Build history of the part. All positions in model axes, mm. A direction names the side the tool comes from. Round coordinates to 2 decimals unless told otherwise and drop trailing zeros. Order: outer loops, then holes, each group sorted by start corner. A loop starts at its lowest first (then second) coordinate and runs counter-clockwise, first axis right, second up. Notation, with made-up numbers: (46, 27.25) -> (80, 27.25) arc R28 ccw to (80, 66.25) -> close; hole circle Ø1 at (49.25, 70). An arc over 180 degrees is marked (long way). Use a Markdown table: item, result. Add a question column.
Item 1: Slice it at A-A, the plane z = -3.25. Give the cut face in (x, y) (3 decimals).
Item 2: 3-axis set-ups, long thin cutter, end or side, ignore diameter. For faces 4 (the face through (-6, 0, -6.5)), 5 (the face through (0, 0, -3)): which of +Z, -Z, +X, -X, +Y, -Y reach the whole face in a straight line?
Item 3: Slice it at D-D, the plane x = -2.25. Give the cut face in (y, z).
Item 4: Slice it at C-C, the plane x = -5.5. Give the cut face in (y, z), plus the area to 3 significant figures.
Item 5: Probe L1, parallel to X at y = -0.05, z = -4.75; L2, parallel to Y at x = 2.25, z = -1.25; L3, parallel to Z at x = -6.25, y = -0.1. List the from-to ranges inside material, lowest first.
Item 6: Slice it at B-B, the plane y = -0.95. Give the cut face in (x, z) (3 decimals).
Item 7: Two-plate mould, pull along Z, no slides. Class faces 1 (the face through (-5.817, -0.085, -1.697)), 2 (the face through (-8, -1.2, -5)), 3 (the face through (-6, 0, 0)): released by +Z, released by -Z, zero draft, split by the parting line, or undercut.
Item 8: Pin check, flat tip, straight feed: pin 1 (3 mm diameter, centred on x = 1, z = -2.5, fed in from -Y). Stop position of the tip, or through.
Autodesk Inventor part; units mm, degrees
ref_plane "YZ Plane" through (0, 0, 0) normal (1, 0, 0) x (0, 1, 0)
ref_plane "XZ Plane" through (0, 0, 0) normal (0, 1, 0) x (-1, 0, 0)
ref_plane "XY Plane" through (0, 0, 0) normal (0, 0, 1) x (1, 0, 0)
sketch "Sketch1" plane through (0, 0, 0) normal (0, 1, 0) x (-1, 0, 0)
  line L0 (0, 0) -> (10, 0)
  line L1 (10, 0) -> (10, -6.5)
  line L2 (10, -6.5) -> (0, -6.5)
  line L3 (0, -6.5) -> (0, 0)
  arc A0 (0, 0) -> (0, -6.5) centre (0, -3.25) ccw
  dimension "d1" = 6.5
  dimension "d2" = 10
extrude "Extrusion1" add sketch "Sketch1" along normal blind 1
sketch "Sketch2" plane through (0, 0, 0) normal (0, -1, 0) x (1, 0, 0)
  line L0 (-10, -6.5) -> (-10, 0) construction
  line L1 (0, -6.5) -> (-10, -6.5) construction
  arc A0 (0, -6.5) -> (0, 0) centre (0, -3.25) ccw construction
  line L2 (-10, 0) -> (0, 0) construction
  line L3 (-10, 0) -> (-3.5, 0) construction
  line L4 (-3.5, 0) -> (-3.5, -6.5) construction
  line L5 (-3.5, -6.5) -> (-10, -6.5) construction
  line L6 (-10, -6.5) -> (-10, 0) construction
  line L7 (-10, -3.25) -> (-6.625, -3.25) construction
  circle A1 centre (-6.625, -3.25) radius 1.75
  dimension "d5" = 6.5
  dimension "d6" = 3.375
  dimension "d7" = 3.5
extrude "Extrusion2" cut sketch "Sketch2" against normal blind 1
sketch "Sketch3" plane through (0, 0, 0) normal (0, -1, 0) x (1, 0, 0)
  circle A0 centre (-6.625, -3.25) radius 1.75 construction
  line L0 (-10, -6.5) -> (-10, 0) construction
  line L1 (0, -6.5) -> (-10, -6.5) construction
  arc A1 (0, -6.5) -> (0, 0) centre (0, -3.25) ccw construction
  line L2 (-10, 0) -> (0, 0) construction
  circle A2 centre (0, -3.25) radius 3.25 construction
  line L3 (-10, -6.5) -> (-3.5, -6.5)
  line L4 (-3.5, -6.5) -> (-3.5, 0)
  line L5 (-3.5, 0) -> (-10, 0)
  line L6 (-10, 0) -> (-10, -6.5)
  circle A3 centre (-6.625, -3.25) radius 1.75
  dimension "d10" = 6.5
extrude "Extrusion3" add sketch "Sketch3" along normal blind 1.2
properties part number "pinub"
Check sheet entries:
| question | item | result |
|---|---|---|
| 1 | outline | (-10, -1.2) -> (-8.375, -1.2) -> (-8.375, 1) -> (-10, 1) -> close; (-4.875, -1.2) -> (-3.5, -1.2) -> (-3.5, 0) -> (3.25, 0) -> (3.25, 1) -> (-4.875, 1) -> close |
| 2 | face 4 | -Z, +X, -X, +Y, -Y |
| 2 | face 5 | +Z, -Z, +X, -Y |
| 3 | outline | (0, -6.5) -> (1, -6.5) -> (1, 0) -> (0, 0) -> close |
| 4 | outline | (-1.2, -6.5) -> (1, -6.5) -> (1, -4.59) -> (-1.2, -4.59) -> close; (-1.2, -1.91) -> (1, -1.91) -> (1, 0) -> (-1.2, 0) -> close |
| 4 | area | 8.40 mm2 |
| 5 | L1 | -10 to -7.53, -5.72 to -3.5 |
| 5 | L2 | 0 to 1 |
| 5 | L3 | -6.5 to -4.96, -1.54 to 0 |
| 6 | outline | (-10, -6.5) -> (-3.5, -6.5) -> (-3.5, 0) -> (-10, 0) -> close; hole circle Ø3.5 at (-6.625, -3.25) |
| 7 | face 1 | undercut |
| 7 | face 2 | zero draft |
| 7 | face 3 | released by +Z |
| 8 | pin 1 | y = 0 |
